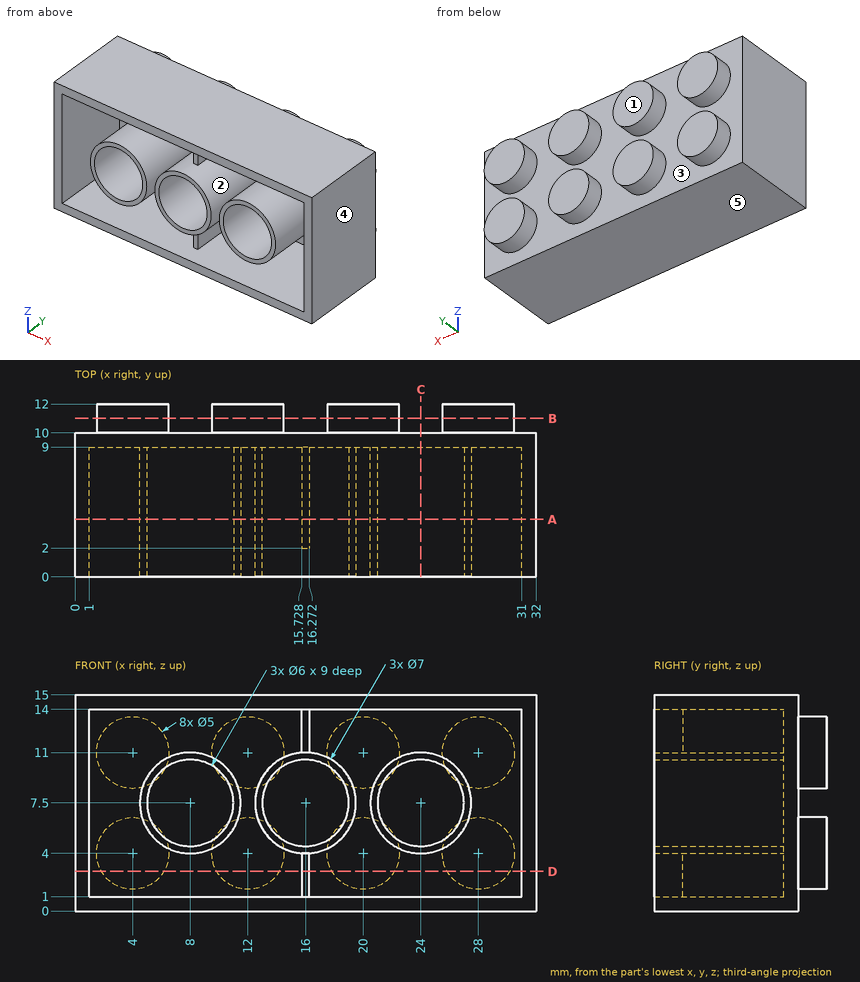
Can you work these out from the drawing? Everything is in mm from the part's minimum corner. A direction names the side the tool comes from. Round coordinates to 2 decimals unless told otherwise and drop trailing zeros. Loops run counter-clockwise (first coordinate to the right, second up) from the corner with the lowest first, then second, coordinate; pieces in that order, holes last. Notation, with made-up numbers: (69, 28.5) - (119, 28.5) arc R16 cw to (119, 48.5) - close; hole circle Ø4 at (44, 32). An arc over 180 degrees is marked (long way). One line per question, with ' | ' between items. Start each with the question number.
Q1. I want a section at B-B (y = 11). Write out the boundary of the cut face in (x, z), then the cut area to 3 significant figures.
Q2. Will these pins go through, and if not, where does the flat tip stop? pin 1 (4.5 mm diameter, centred on x = 23, y = 6, fed in from -Z); pin 2 (5 mm diameter, centred on x = 8, z = 7.5, fed in from +Y); pin 3 (0.6 mm diameter, centred on x = 16, z = 12.5, fed in from -Y); pin 4 (1.8 mm diameter, centred on x = 24, z = 7.5, fed in from -Y).
Q3. For the marked faces 1 and 2, which set-ups out of +Z, -Z, +X, -X, +Y, -Y let a thin tool reach every point of the face, with its end or its side?
Q4. Please list where these lines run through material, in increasing order: line 1 (X direction, y = 4.5, z = 13); line 2 (Z direction, x = 24, y = 6); line 3 (Z direction, x = 30.5, y = 8.75). Write a range as [from, to].
Q5. We'd pull the mould along Z, two halves only. Please class the marked faces 3, 4 and 5: +Z half, -Z half, draft (parallel to the pull), parting line (faces both ways), or undercut.
Q6. I want a section at C-C (x = 24). Write out the boundary of the cut face in (y, z).
Q7. I want a section at A-A (y = 4). Write out the boundary of the cut face in (x, z), then the cut area to 3 significant figures.
Q8. I want a section at D-D (z = 2.75). Write out the boundary of the cut face in (x, y) (1 decimal).
Response values:
1) outline: circle Ø5 at (4, 4); circle Ø5 at (4, 11); circle Ø5 at (12, 4); circle Ø5 at (12, 11); circle Ø5 at (20, 4); circle Ø5 at (20, 11); circle Ø5 at (28, 4); circle Ø5 at (28, 11) | area: 157 mm²
2) pin 1: stops at z = 0 | pin 2: stops at y = 10 | pin 3: stops at y = 2 | pin 4: stops at y = 9
3) face 1: +Z, -Z, +X, -X, +Y | face 2: -Y
4) line 1: x = [0, 1], [15.73, 16.27], [31, 32] | line 2: z = [0, 1], [4, 4.5], [10.5, 11], [14, 15] | line 3: z = [0, 1], [14, 15]
5) face 3: undercut | face 4: draft | face 5: -Z half
6) outline: (0, 0) - (10, 0) - (10, 15) - (0, 15) - (0, 14) - (9, 14) - (9, 11) - (0, 11) - (0, 10.5) - (9, 10.5) - (9, 4.5) - (0, 4.5) - (0, 4) - (9, 4) - (9, 1) - (0, 1) - close
7) outline: (0, 0) - (32, 0) - (32, 15) - (0, 15) - close; circle Ø7 at (8, 7.5); circle Ø7 at (24, 7.5); hole (1, 1) - (15.73, 1) - (15.73, 4.01) arc R3.5 cw to (15.73, 10.99) - (15.73, 14) - (1, 14) - close; hole circle Ø6 at (8, 7.5); hole circle Ø6 at (16, 7.5); hole (16.27, 1) - (31, 1) - (31, 14) - (16.27, 14) - (16.27, 10.99) arc R3.5 cw to (16.27, 4.01) - close; hole circle Ø6 at (24, 7.5) | area: 124 mm²
8) outline: (0, 0) - (1, 0) - (1, 9) - (15.7, 9) - (15.7, 2) - (16.3, 2) - (16.3, 9) - (31, 9) - (31, 0) - (32, 0) - (32, 10) - (30.2, 10) - (30.2, 12) - (25.8, 12) - (25.8, 10) - (22.2, 10) - (22.2, 12) - (17.8, 12) - (17.8, 10) - (14.2, 10) - (14.2, 12) - (9.8, 12) - (9.8, 10) - (6.2, 10) - (6.2, 12) - (1.8, 12) - (1.8, 10) - (0, 10) - close
